Here's how the part is built. I have some questions about the finished solid (model axes, mm). A direction names the side the tool comes from. Coordinates: 2 decimals unless noted, no trailing zeros. Write each loop counter-clockwise with the first axis right and the second up, starting at its lowest first coordinate (ties: lowest second). Pieces come first, ordered by that corner, then holes. Notation, with made-up numbers: M -21.75,0.25 L 21.25,0.25 A11 ccw 21.25,20.25 Z; hole C 79.5,-5.5 d8. An arc over 180 degrees is marked long. Use a Markdown table: item, result.
```python
from build123d import *


# Read off the part's stored shape, not the designer's step: Vaciado1
with BuildPart() as part:
    # Croquis1 → Revolución1 (revolve)
    with BuildSketch(Plane(origin=(0, 0, 0), x_dir=(1, 0, 0), z_dir=(0, 1, 0))):
        Polygon((0, -65), (0, 65), (50, 65), (50, 63), (47.5, 63), (35, 20), (12.5, 5), (12.5, -65), align=None)
    revolve(axis=Axis((0, 0, 65), (0, 0, -1)))

    # Vaciado1 outline → Vaciado1 (revolve, cut)
    with BuildSketch(Plane.XZ):
        Polygon((45.99860382, -65), (33.283256487, -21.259205175), (10.5, -6.070367517), (10.5, 65), (0, 65), (0, -65), align=None)
    revolve(axis=Axis((0, 0, 0), (0, 0, 1)), mode=Mode.SUBTRACT)


solid = part.part
```
1. Will these pins go through, and if not, where does the flat tip stop? pin 1 Ø1 at (x, y) = (-2.5, 30.5) entering from +Z; pin 2 Ø1.5 at (y, z) = (8, -41.5) entering from -X; pin 3 Ø3 at (y, z) = (12, -3.5) entering from -X.
Answers follow:
| item | result |
|---|---|
| pin 1 | stops at z = -16.73 |
| pin 2 | stops at x = -40.73 |
| pin 3 | stops at x = -6.78 |
2. Suppose I cut it at C-C on z = 22. Write out the boundary of the cut face in (x, y), and give its area (3 significant figures).
Answers follow:
| item | result |
|---|---|
| outline | C 0,0 d25; hole C 0,0 d21 |
| area | 145 mm2 |
3. Suppose I cut it at D-D on z = -53.5. Write out the boundary of the cut face in (x, y).
Answers follow:
| item | result |
|---|---|
| outline | C 0,0 d89.48; hole C 0,0 d85.31 |
4. Which directions (+Z, -Z, +X, -X, +Y, -Y) give clear straight access to the entire face, cutting with the end or side of a thin tool? Please do faces 4 (the face through (11.923, -3.755, 30.49)), 5 (the face through (-7.962, -35.853, -33.103)).
Answers follow:
| item | result |
|---|---|
| face 4 | +Z |
| face 5 | -Z |
5. I need wall thicknesses on probe 1 along Y at (x, z) = (0, 35.5); probe 2 along X at (y, z) = (31, -37); probe 3 along X at (y, z) = (-3.5, -45). Which ranges of each line are inside material? Lowest first, please.
Answers follow:
| item | result |
|---|---|
| probe 1 | y = -12.5 to -10.5, 10.5 to 12.5 |
| probe 2 | x = -25.19 to -21.73, 21.73 to 25.19 |
| probe 3 | x = -42.12 to -40.03, 40.03 to 42.12 |
6. Suppose I cut it at A-A on y = 0. Write out the boundary of the cut face in (x, z), and give its area (3 significant figures).
Answers follow:
| item | result |
|---|---|
| outline | M -50,-65 L -46,-65 L -33.28,-21.26 L -10.5,-6.07 L -10.5,65 L -12.5,65 L -12.5,-5 L -35,-20 L -47.5,-63 L -50,-63 Z; M 10.5,-6.07 L 33.28,-21.26 L 46,-65 L 50,-65 L 50,-63 L 47.5,-63 L 35,-20 L 12.5,-5 L 12.5,65 L 10.5,65 Z |
| area | 585 mm2 |
7. We'd pull the mould along Y, two halves only. Please class faces 1 (the face through (47.69, -15.02, -63.99)), 2 (the face through (-9.21, -7.062, -6.808)), 3 (the face through (44.2, 18.3, -63)): +Y half, -Y half, draft (parallel to the pull), parting line (faces both ways), or undercut.
Answers follow:
| item | result |
|---|---|
| face 1 | parting line |
| face 2 | undercut |
| face 3 | draft |
